For this review, take the finished solid that the model builds, in its own axes (mm). A direction names the side the tool comes from. Give positions to 0.01 mm unless a question says otherwise; leave off trailing zeros. Loops run counter-clockwise (first coordinate to the right, second up) from the corner with the lowest first, then second, coordinate; pieces in that order, holes last.
```python
from build123d import *

# Parameters (mm, degrees)
F0_R         = 4
F0_R_2       = 1.5
F1_DEPTH     = 5
F0_W         = 86
F0_H         = 66
F2_DEPTH     = 2
F0_W_2       = 90
F0_H_2       = 70
F3_DEPTH     = 30
F4_R         = 1.5
F5_DEPTH     = 2
F6_R         = 3
F6_R_2       = 1.5
F7_DEPTH     = 0.75
F9_W         = 5
F9_H         = 5
F10_DEPTH    = 8
F11_C1_SIZE  = 3
F11_C2_SIZE  = 3
F11_C3_SIZE  = 3
F11_C4_SIZE  = 3
F12_SIZE     = 2
F13_W        = 78
F13_H        = 9
F14_DEPTH    = 2
F15_SIZE     = 4
F16_T1_DEPTH = 2
F17_W        = 5
F17_H        = 2
F18_DEPTH    = 9
F19_SIZE     = 0.8
F9_H_2       = 8
F9_R         = 1.5
F20_DEPTH    = 15
F21_T4_DEPTH = 59.7965774757
F21_T9_DEPTH = 59.7965774757


# Not quite as in the source:
# - a fillet or chamfer that OpenCascade refuses, or shapes differently, is made with other operations: its cross-section is extruded or revolved along the edge and cut away or added
# - two fillets or chamfers of one size are made in one step


with BuildPart() as f1:
    # F0 (on Top) → F1 (new body)
    with BuildSketch(Plane.XY):
        with Locations((-35, 21.5)):
            Circle(F0_R)
        with Locations((-35, 21.5)):
            Circle(F0_R_2, mode=Mode.SUBTRACT)
    extrude(amount=F1_DEPTH)



with BuildPart() as f1b:
    # F0 (on Top) → F1, piece 2 (new body)
    with BuildSketch(Plane.XY):
        with Locations((35, 21.5)):
            Circle(F0_R)
        with Locations((35, 21.5)):
            Circle(F0_R_2, mode=Mode.SUBTRACT)
    extrude(amount=F1_DEPTH)


with BuildPart() as f1c:
    # F0 (on Top) → F1, piece 3 (new body)
    with BuildSketch(Plane.XY):
        with Locations((35, -21.5)):
            Circle(F0_R)
        with Locations((35, -21.5)):
            Circle(F0_R_2, mode=Mode.SUBTRACT)
    extrude(amount=F1_DEPTH)


with BuildPart() as f1d:
    # F0 (on Top) → F1, piece 4 (new body)
    with BuildSketch(Plane.XY):
        with Locations((-35, -21.5)):
            Circle(F0_R)
        with Locations((-35, -21.5)):
            Circle(F0_R_2, mode=Mode.SUBTRACT)
    extrude(amount=F1_DEPTH)


with BuildPart() as f1_1:
    add(f1.part)

    add(f1b.part)  # F2 merges F1b

    add(f1c.part)  # F2 merges F1c

    add(f1d.part)  # F2 merges F1d
    # F0 (on Top) → F2 (join)
    with BuildSketch(Plane.XY):
        Rectangle(F0_W, F0_H)
        with Locations((-35, -21.5)):
            Circle(F0_R, mode=Mode.SUBTRACT)
        with Locations((35, -21.5)):
            Circle(F0_R, mode=Mode.SUBTRACT)
        with Locations((-35, 21.5)):
            Circle(F0_R, mode=Mode.SUBTRACT)
        with Locations((35, 21.5)):
            Circle(F0_R, mode=Mode.SUBTRACT)
        with Locations((-35, 21.5)):
            Circle(F0_R)
        with Locations((-35, 21.5)):
            Circle(F0_R_2, mode=Mode.SUBTRACT)
        with Locations((35, 21.5)):
            Circle(F0_R_2)
        with Locations((35, -21.5)):
            Circle(F0_R_2)
        with Locations((-35, -21.5)):
            Circle(F0_R_2)
        with Locations((-35, 21.5)):
            Circle(F0_R_2)
    extrude(amount=F2_DEPTH)

    # F0 (on Top) → F3 (join)
    with BuildSketch(Plane.XY):
        Rectangle(F0_W_2, F0_H_2)
        Rectangle(F0_W, F0_H, mode=Mode.SUBTRACT)
    extrude(amount=F3_DEPTH)

    # F4 (on face) → F5 (cut, through all)
    with BuildSketch(Plane.XZ.offset(35)):
        with Locations((-30, 10)):
            Circle(F4_R)
        with Locations((0, 10)):
            Circle(F4_R)
        with Locations((30, 10)):
            Circle(F4_R)
    extrude(amount=-F5_DEPTH, mode=Mode.SUBTRACT)

    # F6 (on face) → F7 (cut)
    with BuildSketch(Plane(origin=(0, -33, 0), x_dir=(-1, 0, 0), z_dir=(0, 1, 0))):
        with Locations((-30, 10)):
            Circle(F6_R)
        with Locations((-30, 10)):
            Circle(F6_R_2, mode=Mode.SUBTRACT)
        with Locations((0, 10)):
            Circle(F6_R)
        with Locations((0, 10)):
            Circle(F6_R_2, mode=Mode.SUBTRACT)
        with Locations((30, 10)):
            Circle(F6_R)
        with Locations((30, 10)):
            Circle(F6_R_2, mode=Mode.SUBTRACT)
    extrude(amount=-F7_DEPTH, mode=Mode.SUBTRACT)

    # F9 (on offset) → F10 (join)
    with BuildSketch(Plane.XY.offset(26)):
        with Locations((40.5, -30.5)):
            Rectangle(F9_W, F9_H)
        with Locations((40.5, 30.5)):
            Rectangle(F9_W, F9_H)
        with Locations((-40.5, -30.5)):
            Rectangle(F9_W, F9_H)
        with Locations((-40.5, 30.5)):
            Rectangle(F9_W, F9_H)
    extrude(amount=-F10_DEPTH)

    # F11: chamfer of 3 on 4 edges, made by hand

    # F11_c1
    f11_c1_edges = [f1_1.edges().sort_by_distance(p)[0] for p in [
        (-38, -30.5, 18),
    ]]
    chamfer(f11_c1_edges, length=F11_C1_SIZE)

    # F11_c2
    f11_c2_edges = [f1_1.edges().sort_by_distance(p)[0] for p in [
        (38, -30.5, 18),
    ]]
    chamfer(f11_c2_edges, length=F11_C2_SIZE)

    # F11_c3
    f11_c3_edges = [f1_1.edges().sort_by_distance(p)[0] for p in [
        (-38, 30.5, 18),
    ]]
    chamfer(f11_c3_edges, length=F11_C3_SIZE)

    # F11_c4
    f11_c4_edges = [f1_1.edges().sort_by_distance(p)[0] for p in [
        (38, 30.5, 18),
    ]]
    chamfer(f11_c4_edges, length=F11_C4_SIZE)

    # F12
    f12_edges = [f1_1.edges().sort_by_distance(p)[0] for p in [
        (-38, 28, 23.5),
        (-38, -28, 23.5),
        (38, -28, 23.5),
        (38, 28, 23.5),
    ]]
    chamfer(f12_edges, length=F12_SIZE)

    # F13 (on face) → F14 (cut, through all)
    with BuildSketch(Plane(origin=(0, 35, 0), x_dir=(-1, 0, 0), z_dir=(0, 1, 0))):
        with Locations((0, 10.5)):
            Rectangle(F13_W, F13_H)
    extrude(amount=-F14_DEPTH, mode=Mode.SUBTRACT)

    # F15
    f15_edges = [f1_1.edges().sort_by_distance(p)[0] for p in [
        (-39, 34, 15),
        (39, 34, 15),
    ]]
    chamfer(f15_edges, length=F15_SIZE)

    # F16: fillet of radius 4 on 6 edges, made by hand

    # F16_s2 → F16_t1 (join)
    with BuildSketch(Plane.XZ.offset(-35)):
        with BuildLine():
            ThreePointArc((-39, 10), (-37.8284271247, 7.1715728753), (-35, 6))
            Line((-35, 6), (-39, 6))
            Line((-39, 6), (-39, 10))
        make_face()
        with BuildLine():
            ThreePointArc((39, 10), (37.8284271247, 7.1715728753), (35, 6))
            Line((35, 6), (39, 6))
            Line((39, 6), (39, 10))
        make_face()
        with BuildLine():
            ThreePointArc((-33.3431457505, 15), (-34.87387948, 14.69551813), (-36.1715728753, 13.8284271247))
            Line((-36.1715728753, 13.8284271247), (-35, 15))
            Line((-35, 15), (-33.3431457505, 15))
        make_face()
        with BuildLine():
            ThreePointArc((33.3431457505, 15), (34.87387948, 14.69551813), (36.1715728753, 13.8284271247))
            Line((36.1715728753, 13.8284271247), (35, 15))
            Line((35, 15), (33.3431457505, 15))
        make_face()
        with BuildLine():
            ThreePointArc((-37.8284271247, 12.1715728753), (-38.69551813, 10.87387948), (-39, 9.3431457505))
            Line((-39, 9.3431457505), (-39, 11))
            Line((-39, 11), (-37.8284271247, 12.1715728753))
        make_face()
        with BuildLine():
            ThreePointArc((37.8284271247, 12.1715728753), (38.69551813, 10.87387948), (39, 9.3431457505))
            Line((39, 9.3431457505), (39, 11))
            Line((39, 11), (37.8284271247, 12.1715728753))
        make_face()
    extrude(amount=F16_T1_DEPTH)

    # F17 (on face) → F18 (join, through all)
    with BuildSketch(Plane(origin=(0, 0, 15), x_dir=(1, 0, 0), z_dir=(0, 0, -1))):
        with Locations((0, -34)):
            Rectangle(F17_W, F17_H)
    extrude(amount=F18_DEPTH)

    # F19
    f19_edges = [f1_1.edges().sort_by_distance(p)[0] for p in [
        (2.5, 35, 10.5),
        (-2.5, 35, 10.5),
        (2.5, 33, 10.5),
        (-2.5, 33, 10.5),
    ]]
    chamfer(f19_edges, length=F19_SIZE)

    # F9 (on offset) → F20 (join)
    with BuildSketch(Plane.XY.offset(26)):
        with Locations((-40.5, 0)):
            Rectangle(F9_W, F9_H_2)
        with Locations((-41, 0)):
            Circle(F9_R, mode=Mode.SUBTRACT)
        with Locations((40.5, 0)):
            Rectangle(F9_W, F9_H_2)
        with Locations((41, 0)):
            Circle(F9_R, mode=Mode.SUBTRACT)
    extrude(amount=-F20_DEPTH)

    # F21: chamfer of 5 x 10 on 2 edges, made by hand


with BuildPart() as f21_tool2:
    # F21_s3 → F21_t4 (new body)
    with BuildSketch(Plane.XZ.offset(-29.8982887379)):
        Polygon((38, 21), (43, 11), (38, 11), align=None)
    extrude(amount=F21_T4_DEPTH)

    split(bisect_by=Plane.YZ.offset(43), keep=Keep.BOTTOM)


with BuildPart() as f1_2:
    add(f1_1.part)

    # F21_t1: cut F21_tool2
    add(f21_tool2.part, mode=Mode.SUBTRACT)


with BuildPart() as f21_tool7:
    # F21_s8 → F21_t9 (new body)
    with BuildSketch(Plane.XZ.offset(29.8982887379)):
        Polygon((-38, 21), (-43, 11), (-38, 11), align=None)
    extrude(amount=-F21_T9_DEPTH)

    split(bisect_by=Plane.YZ.offset(-43), keep=Keep.TOP)


with BuildPart() as f1_3:
    add(f1_2.part)

    # F21_t6: cut F21_tool7
    add(f21_tool7.part, mode=Mode.SUBTRACT)


solid = f1_3.part
```
Q1. Consider section D-D on x = 0. Give the boundary of the cut face in (y, z).
Answers:
outline: (-35, 0) - (35, 0) - (35, 30) - (33, 30) - (33, 2) - (-33, 2) - (-33, 7) - (-33.75, 7) - (-33.75, 8.5) - (-35, 8.5) - close; (-35, 11.5) - (-33.75, 11.5) - (-33.75, 13) - (-33, 13) - (-33, 30) - (-35, 30) - close
Q2. For probe 1 along X at (y, z) = (-34.1, 10); probe 2 along X at (y, z) = (31, 27); probe 3 along Y at (x, z) = (-23.5, 19), list the stretches that pass through material, from the lowest coordinate up.
Answers:
probe 1: x = -45 to -31.5, -28.5 to -1.5, 1.5 to 28.5, 31.5 to 45
probe 2: x = -45 to -43, 43 to 45
probe 3: y = -35 to -33, 33 to 35
Q3. Consider section B-B on y = 0. Give the boundary of the cut face in (x, z), plus the area to 3 significant figures.
Answers:
outline: (-45, 0) - (45, 0) - (45, 30) - (43, 30) - (43, 26) - (42.5, 26) - (42.5, 12) - (43, 11) - (43, 2) - (-43, 2) - (-43, 11) - (-42.5, 12) - (-42.5, 26) - (-43, 26) - (-43, 30) - (-45, 30) - close; (-39.5, 18) - (-38, 21) - (-38, 26) - (-39.5, 26) - close; (38, 21) - (39.5, 18) - (39.5, 26) - (38, 26) - close
area: 326 mm2
Q4. Consider section C-C on z = 23.5. Count the separate pieces of the cut face and the enclosed holes in it, plus the area to 3 significant figures.
Answers:
separate pieces: 1
enclosed holes: 3
area: 782 mm2
Q5. Mouldability with a two-part tool opening along Z and no side actions: class faces 6 (the flat face through (41, 28, 22)), 7 (the flat face through (42, 31, 18)), 8 (the flat face through (-35, 22, 2)), 9 (the flat face through (18, 34, 15)) as +Z half, -Z half, draft (parallel to the pull), parting line (faces both ways), or undercut.
Answers:
face 6: draft
face 7: undercut
face 8: +Z half
face 9: undercut
Q6. Consider section A-A on x = -30. Give the boundary of the cut face in (y, z), plus the area to 3 significant figures.
Answers:
outline: (-35, 0) - (35, 0) - (35, 6) - (33, 6) - (33, 2) - (-33, 2) - (-33, 7) - (-33.75, 7) - (-33.75, 8.5) - (-35, 8.5) - close; (-35, 11.5) - (-33.75, 11.5) - (-33.75, 13) - (-33, 13) - (-33, 30) - (-35, 30) - close; (33, 15) - (35, 15) - (35, 30) - (33, 30) - close
area: 226 mm2
Q7. For pin 1 Ø4 at (x, y) = (17.5, 14) entering from +Z; pin 2 Ø1.5 at (x, y) = (40.5, -30.5) entering from +Z; pin 3 Ø6.5 at (x, z) = (-30, 9.5) entering from +Y, all flat-tipped, find the tip position at first contact; note any pin that passes through.
Answers:
pin 1: stops at z = 2
pin 2: stops at z = 26
pin 3: stops at y = -33
Q8. Machinability: for faces 1 (the flat face through (-42, 28, 22)), 2 (the cylindrical face through (28.5, -34.38, 10.07)), 3 (the flat face through (-42, -30, 18)), 4 (the flat face through (-1, -35, 15)), 5 (the cylindrical face through (-38.621, 34.014, 11.042)), which of the approach directions +Z, -Z, +X, -X, +Y, -Y give a long, thin tool a straight path to every point of the face, cutting with its end or side? Answer none if there is none.
Answers:
face 1: +Z
face 2: +Y, -Y
face 3: none
face 4: +Z, -Z, +X, -X, -Y
face 5: +Y
